Source: CAD feature listing. Evaluate the final solid. Frame: model axes, mm. Face numbers are marked on the shaded views. A direction names the side the tool comes from. Coordinates: 2 decimals unless noted, no trailing zeros. Write each loop counter-clockwise with the first axis right and the second up, starting at its lowest first coordinate (ties: lowest second). Pieces come first, ordered by that corner, then holes. Notation, with made-up numbers: M 37.5,-17 L 68.5,-17 A18 cw 68.5,13 Z; hole C 60,39.25 d9. An arc over 180 degrees is marked long. One line per item, written item: value. Start each with the question number.
Item 1: Mould query, pull axis X, two halves, no side actions, for the marked faces 4, 5, 6 and 7. Classes: released by +X, released by -X, zero draft, split by the parting line, or undercut.
Item 2: Cut plane A-A, the plane x = -95.5. Output: boundary loops of the cut face in (y, z), then the cut area to 3 significant figures.
Item 3: Ray query, L1, parallel to Z at x = -96.75, y = 15; L2, parallel to X at y = -13.5, z = -8; L3, parallel to X at y = 18, z = 1.5. Return the intervals inside material, ascending. Write a range as from..to.
Item 4: Set-up query: the marked faces 1, 2 and 3. Return all of +Z, -Z, +X, -X, +Y, -Y with unobstructed straight access to the full face (end or side cutting, diameter ignored); none if empty.
Item 5: Cut plane B-B, the plane x = -58. Output: boundary loops of the cut face in (y, z), then the cut area to 3 significant figures.
Item 6: Pin query (flat end, axial travel): P1, Ø3.5, axis at y = 0, z = 15, coming from the -X side; P2, Ø12, axis at y = -15, z = -8.5, coming from the -X side; P3, Ø5, axis at x = -74, z = 12, coming from the +Y side. Return the tip coordinate at first contact, or that it passes through.
```python
from build123d import *
from build123d.topology import SkipClean

# Parameters (mm, degrees)
SKETCH2_R           = 1.5
CUT_EXTRUDE1_DEPTH  = 8
CHAMFER1_SIZE       = 0.5
BOSS_EXTRUDE1_DEPTH = 12
CUT_EXTRUDE2_START  = -5
CUT_EXTRUDE2_DEPTH  = 5


with BuildPart() as part:
    # Sketch1 → Revolve1 (revolve)
    with BuildSketch(Plane.XY):
        Polygon((-120.1, 0), (-120.1, 3.5), (-119.6, 4), (-102.1, 4), (-102.1, 9.3), (-101.9, 9.5), (-102.1, 9.7), (-102.1, 10.8), (-101.9, 11), (-100.1, 11), (-100.1, 17.8), (-99.9, 18), (-91.8, 18), (-91.4, 17.6), (-91.4, 17.5), (-70.2, 17.5), (-70.2, 17.6), (-69.8, 18), (-65.6, 18), (-65.2, 17.6), (-64.8, 18), (-61.4, 18), (-61.2, 17.8), (-61, 18), (-6.2, 18), (-6, 17.8), (-5.8, 18), (-3.4, 18), (-3, 17.6), (-2.6, 18), (-0.4, 18), (0, 17.6), (0, 0), align=None)
    revolve(axis=Axis((0, 0, 0), (-1, 0, 0)))

    # Sketch2 → Cut-Extrude1 (cut)
    with BuildSketch(Plane.ZY.offset(100.1)):
        with Locations(Location((-15, 0, 0), (0, 0, 270))):
            Circle(SKETCH2_R)
        with Locations(Location((0, 15, 0), (0, 0, 270))):
            Circle(SKETCH2_R)
        with Locations(Location((15, 0, 0), (0, 0, 270))):
            Circle(SKETCH2_R)
        with Locations(Location((0, -15, 0), (0, 0, 270))):
            Circle(SKETCH2_R)
    extrude(amount=-CUT_EXTRUDE1_DEPTH, mode=Mode.SUBTRACT)

    # Chamfer1
    chamfer1_edges = [part.edges().sort_by_distance(p)[0] for p in [
        (-100.1, 1.5, -15),
        (-100.1, 16.5, 0),
        (-100.1, 1.5, 15),
        (-100.1, -13.5, 0),
    ]]
    chamfer(chamfer1_edges, length=CHAMFER1_SIZE)

    # Sketch3 → Boss-Extrude1 (add)
    with BuildSketch(Plane(origin=(0, 0, 0), x_dir=(0, 0, -1), z_dir=(1, 0, 0))):
        with BuildLine():
            Line((18.2, 21.8), (-10.8, 21.8))
            Line((-10.8, 21.8), (-14.2, 17.8))
            Line((-14.2, 17.8), (-18.2, 17.8))
            Line((-18.2, 17.8), (-18.2, 0))
            ThreePointArc((-18.2, 0), (-13.72479508, -11.952823934), (-2.5, -18.027479025))
            Line((-2.5, -18.027479025), (-2.5, -19.027479025))
            ThreePointArc((-2.5, -19.027479025), (0, -20.2), (2.5, -19.027479025))
            Line((2.5, -19.027479025), (2.5, -18.027479025))
            ThreePointArc((2.5, -18.027479025), (13.72479508, -11.952823934), (18.2, 0))
            Line((18.2, 0), (18.2, 21.8))
        make_face()
    extrude(amount=BOSS_EXTRUDE1_DEPTH)

    # Sketch4 → Cut-Extrude2 (cut)
    with SkipClean():  # the faces are left unmerged after this step: merging them gives an invalid solid
        with BuildSketch(Plane(origin=(12, 0, 0), x_dir=(0, 0, -1), z_dir=(1, 0, 0)).offset(CUT_EXTRUDE2_START)):
            with BuildLine():
                Line((2.5, -19.027479025), (2.5, -18.027479025))
                ThreePointArc((2.5, -18.027479025), (0, -18.2), (-2.5, -18.027479025))
                Line((-2.5, -18.027479025), (-2.5, -19.027479025))
                ThreePointArc((-2.5, -19.027479025), (0, -20.2), (2.5, -19.027479025))
            make_face()
        extrude(amount=CUT_EXTRUDE2_DEPTH, mode=Mode.SUBTRACT)


solid = part.part
```
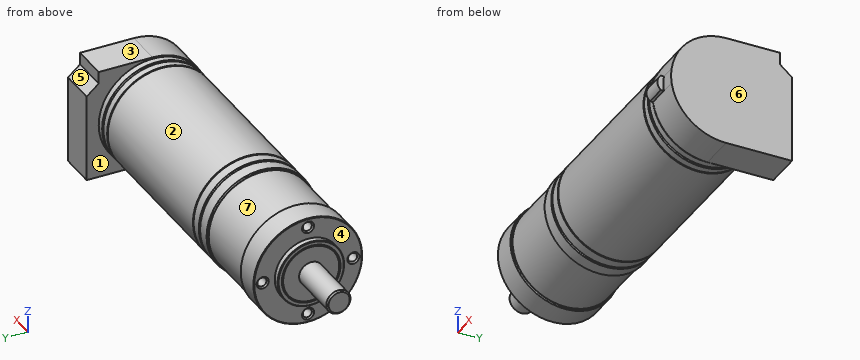
From the geometry:
1. face 4: released by -X
1. face 5: zero draft
1. face 6: released by +X
1. face 7: undercut
2. outline: C 0,0 d36; hole C -15,0 d3; hole C 0,-15 d3; hole C 0,15 d3; hole C 15,0 d3
2. area: 990 mm²
3. L1: z = -9.95..-1.5, 1.5..9.95
3. L2: x = -100.1..12
3. L3: x = 0..12
4. face 1: none
4. face 2: -X
4. face 3: +Z, +X, -X, +Y, -Y
5. outline: C 0,0 d36
5. area: 1,020 mm²
6. P1: stops at x = -99.85
6. P2: stops at x = -100.1
6. P3: stops at y = 14.7
